Design review of the part built by this model. Coordinates are the model's own, in mm. A direction names the side the tool comes from. Coordinates: 2 decimals unless noted, no trailing zeros. Write each loop counter-clockwise with the first axis right and the second up, starting at its lowest first coordinate (ties: lowest second). Pieces come first, ordered by that corner, then holes. Notation, with made-up numbers: (70, 8) -> (126, 8) arc R16 ccw to (126, 24) -> close; hole circle Ø6 at (12, 16.5). An arc over 180 degrees is marked (long way). Return JSON: item names as keys, results as strings. Group by question number.
from build123d import *

# Parameters (mm, degrees)
F1_DEPTH = 63.5
F0_W     = 25.4
F0_H     = 19.05
F0_H_2   = 7.4700546124
F0_H_3   = 2.0549453876
F2_DEPTH = 25.4
F3_DEPTH = 7.9375


with BuildPart() as f1:
    # F0 (on Front) → F1 (new body, symmetric)
    with BuildSketch(Plane.XZ):
        Polygon((-41.275, -9.525), (41.275, -9.525), (41.275, 9.525), (22.225, 9.525), (-41.275, 9.525), align=None)
    extrude(amount=F1_DEPTH, both=True)

    # F0 (on Front) → F2 (join, symmetric)
    with BuildSketch(Plane.XZ):
        with BuildLine():
            Line((22.225, 9.525), (41.275, 9.525))
            Line((41.275, 9.525), (41.275, 29.6950546124))
            ThreePointArc((41.275, 29.6950546124), (45.9246798487, 40.9203747637), (57.15, 45.5700546124))
            Line((57.15, 45.5700546124), (60.325, 45.5700546124))
            Line((60.325, 45.5700546124), (60.325, 64.6200546124))
            Line((60.325, 64.6200546124), (57.15, 64.6200546124))
            ThreePointArc((57.15, 64.6200546124), (32.4542956671, 54.3907589453), (22.225, 29.6950546124))
            Line((22.225, 29.6950546124), (22.225, 9.525))
        make_face()
        Polygon((85.725, 66.675), (85.725, 64.6200546124), (85.725, 45.5700546124), (85.725, 38.1), (111.125, 38.1), (111.125, 66.675), align=None)
        with Locations((73.025, 55.0950546124)):
            Rectangle(F0_W, F0_H)
        with Locations((73.025, 41.8350273062)):
            Rectangle(F0_W, F0_H_2)
        with Locations((73.025, 65.6475273062)):
            Rectangle(F0_W, F0_H_3)
    extrude(amount=F2_DEPTH, both=True)

    # F0 (on Front) → F3 (join, symmetric)
    with BuildSketch(Plane.XZ):
        with BuildLine():
            add(Edge.make_bspline(
                [(-41.275, 9.525), (-9.4534000382, 48.0157919228), (16.3796581328, 66.3610100746), (57.15, 64.6200546124)],
                knots=[0, 0, 0, 0, 112.7960356916, 112.7960356916, 112.7960356916, 112.7960356916], degree=3))
            Line((-41.275, 9.525), (22.225, 9.525))
            Line((22.225, 9.525), (22.225, 29.6950546124))
            ThreePointArc((22.225, 29.6950546124), (32.4542956671, 54.3907589453), (57.15, 64.6200546124))
        make_face()
    extrude(amount=F3_DEPTH, both=True)


solid = f1.part
Q1. We need section A-A on z = -4. Write out the cut boundary in (x, y) (3 decimals), plus the area to 3 significant figures.
Q2. For P1, Ø15, axis at x = 87, y = 11, coming from the -Z side; P2, Ø3.5, axis at y = -2.5, z = 43, coming from the -X side; P3, Ø17, axis at x = 62.5, z = 52, coming from the -Y side; P4, Ø1, axis at y = -26.5, z = 17.5, coming from the -X side, all flat-tipped, find the tip position at first contact; note any pin that passes through.
Q3. For faces 1 (the flat face through (60.325, 0, 42)), 2 (the flat face through (66, -25.4, 45)), 3 (the flat face through (85, 0, 38.1)), 4 (the flat face through (9, -7.938, 32)), list the 3-axis set-ups (+Z, -Z, +X, -X, +Y, -Y) from which the entire face can be reached by the end or side of a thin tool; tool diameter is ignored.
Q4. Wall thickness on L1, parallel to Z at x = -9.5, y = 48.5 (3 decimals); L2, parallel to Y at x = -21, z = 14.5; L3, parallel to X at y = 10, z = -4 (3 decimals): over which ranges is each line inside the solid? List them lowest first.
Q5. We need section B-B on x = 64. Write out the cut boundary in (y, z) (3 decimals).
Findings below:
{
 "1": {"outline": "(-41.275, -63.5) -> (41.275, -63.5) -> (41.275, 63.5) -> (-41.275, 63.5) -> close", "area": "10,500 mm^2"},
 "2": {"P1": "stops at z = 38.1", "P2": "stops at x = -10.74", "P3": "stops at y = -25.4", "P4": "passes through"},
 "3": {"face 1": "-Z, +Y, -Y", "face 2": "+Z, +X, -X, -Y", "face 3": "-Z, +X, +Y, -Y", "face 4": "+Z, -X, -Y"},
 "4": {"L1": "z = -9.525 to 9.525", "L2": "y = -7.94 to 7.94", "L3": "x = -41.275 to 41.275"},
 "5": {"outline": "(-25.4, 38.1) -> (25.4, 38.1) -> (25.4, 66.675) -> (-25.4, 66.675) -> close"}
}
